CAD build for the part. Positions are in the model's coordinates, mm. Coordinates: 2 decimals unless noted, no trailing zeros. Loops run counter-clockwise (first coordinate to the right, second up) from the corner with the lowest first, then second, coordinate; pieces in that order, holes last. Notation, with made-up numbers: (66, 5.25) -> (85, 5.25) arc R37 cw to (85, 43.25) -> close; hole circle Ø1 at (-10.75, -3.5). An arc over 180 degrees is marked (long way). Answer as CSV lines item,"result". Start each with the question number.
from build123d import *

# Parameters (mm, degrees)
SKETCH_1_W      = 20
SKETCH_1_H      = 28
SKETCH_1_R      = 2.05
SKETCH_1_R_2    = 3.1
EXTRUDE_2_DEPTH = 5
FILLET_1_R      = 2


with BuildPart() as part:
    # 草图1 → 凸台-拉伸2 (new, symmetric)
    with BuildSketch(Plane.XY):
        Rectangle(SKETCH_1_W, SKETCH_1_H)
        with Locations((0, 10)):
            Circle(SKETCH_1_R, mode=Mode.SUBTRACT)
        with Locations((0, -10)):
            Circle(SKETCH_1_R, mode=Mode.SUBTRACT)
        Circle(SKETCH_1_R_2, mode=Mode.SUBTRACT)
    extrude(amount=EXTRUDE_2_DEPTH, both=True)

    # 圆角1
    fillet_1_edges = [part.edges().sort_by_distance(p)[0] for p in [
        (10, -14, 0),
        (-10, -14, 0),
        (-10, 14, 0),
        (10, 14, 0),
    ]]
    fillet(fillet_1_edges, radius=FILLET_1_R)


solid = part.part
Item 1: Saw through at B-B (z = -4.5). Write the cut outline in (x, y).
Item 2: Saw through at A-A (x = 0). Write the cut outline in (y, z), plus the area to 3 significant figures.
Item 3: Saw through at C-C (y = 0). Write the cut outline in (x, z).
Item 4: Wall check: probe 1 along Y at (x, z) = (0, 2.25); probe 2 along Y at (x, z) = (1, 1); probe 3 along X at (y, z) = (8.75, 1.25). Give the ranges that are in metal, low to high.
Item 5: Two-plate mould, pull along X, no slides. Class faces 1 (the face through (10, 0, 0)), 2 (the face through (-0.444, -12.001, -0.07)), 3 (the face through (-9.43, 13.4, -0.07)): pulls with the +X half, pulls with the -X half, needs draft (parallel to the pull), parting line crosses it, or undercut.
Item 6: Saw through at D-D (y = -10). Write the cut outline in (x, z), plus the area to 3 significant figures.
Geometry check:
1,outline,"(-10, -12) arc R2 ccw to (-8, -14) -> (8, -14) arc R2 ccw to (10, -12) -> (10, 12) arc R2 ccw to (8, 14) -> (-8, 14) arc R2 ccw to (-10, 12) -> close; hole circle Ø6.2 at (0, 0); hole circle Ø4.1 at (0, -10); hole circle Ø4.1 at (0, 10)"
2,outline,"(-14, -5) -> (-12.05, -5) -> (-12.05, 5) -> (-14, 5) -> close; (-7.95, -5) -> (-3.1, -5) -> (-3.1, 5) -> (-7.95, 5) -> close; (3.1, -5) -> (7.95, -5) -> (7.95, 5) -> (3.1, 5) -> close; (12.05, -5) -> (14, -5) -> (14, 5) -> (12.05, 5) -> close"
2,area,"136 mm2"
3,outline,"(-10, -5) -> (-3.1, -5) -> (-3.1, 5) -> (-10, 5) -> close; (3.1, -5) -> (10, -5) -> (10, 5) -> (3.1, 5) -> close"
4,probe 1,"-14 to -12.05, -7.95 to -3.1, 3.1 to 7.95, 12.05 to 14"
4,probe 2,"-14 to -11.79, -8.21 to -2.93, 2.93 to 8.21, 11.79 to 14"
4,probe 3,"-10 to -1.62, 1.62 to 10"
5,face 1,"pulls with the +X half"
5,face 2,"undercut"
5,face 3,"pulls with the -X half"
6,outline,"(-10, -5) -> (-2.05, -5) -> (-2.05, 5) -> (-10, 5) -> close; (2.05, -5) -> (10, -5) -> (10, 5) -> (2.05, 5) -> close"
6,area,"159 mm2"
